from build123d import *

# Parameters (mm, degrees)
SKETCH_1_R          = 2.5
EXTRUDE_1_DEPTH     = 3
CUT_EXTRUDE_1_DEPTH = 2
SKETCH_3_R          = 1.5
EXTRUDE_2_DEPTH     = 10
FILLET_1_R          = 0.5
SKETCH_4_R          = 1.5
EXTRUDE_3_DEPTH     = 2


with BuildPart() as part:
    # 草图1 → 凸台-拉伸1 (new body)
    with BuildSketch(Plane(origin=(0, 0, 0), x_dir=(1, 0, 0), z_dir=(0, 1, 0))):
        with Locations(Location((0, 0, 0), (0, 0, 270))):
            Circle(SKETCH_1_R)
    extrude(amount=EXTRUDE_1_DEPTH)

    # 草图2 → 切除-拉伸1 (cut)
    with BuildSketch(Plane(origin=(0, 3, 0), x_dir=(1, 0, 0), z_dir=(0, 1, 0))):
        Polygon((0, 1.5), (-1.299038106, 0.75), (-1.299038106, -0.75), (0, -1.5), (1.299038106, -0.75), (1.299038106, 0.75), align=None)
    extrude(amount=-CUT_EXTRUDE_1_DEPTH, mode=Mode.SUBTRACT)

    # 草图3 → 凸台-拉伸2 (add)
    with BuildSketch(Plane.XZ):
        with Locations(Location((0, 0, 0), (0, 0, 270))):
            Circle(SKETCH_3_R)
    extrude(amount=EXTRUDE_2_DEPTH)

    # 圆角1
    fillet_1_edges = [part.edges().sort_by_distance(p)[0] for p in [
        (0, 0, -2.5),
        (0, 3, -2.5),
    ]]
    fillet(fillet_1_edges, radius=FILLET_1_R)

    # 草图4 → 凸台-拉伸3 (add)
    with BuildSketch(Plane.XZ.offset(10)):
        with Locations(Location((0, 0, 0), (0, 0, 270))):
            Circle(SKETCH_4_R)
    extrude(amount=EXTRUDE_3_DEPTH)


solid = part.part
Source: CAD feature listing. Evaluate the final solid. Frame: model axes, mm. A direction names the side the tool comes from. Round coordinates to 2 decimals unless told otherwise and drop trailing zeros. Loops run counter-clockwise (first coordinate to the right, second up) from the corner with the lowest first, then second, coordinate; pieces in that order, holes last. Notation, with made-up numbers: M 44,57 L 62,57 A23 ccw 62,65 Z; hole C 2.25,55 d3. An arc over 180 degrees is marked long. Return JSON: item names as keys, results as strings. Group by question number.
1. Section query A-A on z = 0. Output: boundary loops of the cut face in (x, y), and give its area (3 significant figures).
2. Pin query (flat end, axial travel): pin 1 (1.6 mm diameter, centred on y = 2.5, z = -0.5, fed in from +X); pin 2 (1 mm diameter, centred on x = 0.5, y = -6.5, fed in from +Z); pin 3 (1.5 mm diameter, centred on y = -7.5, z = 1.5, fed in from +X). Return the tip coordinate at first contact, or that it passes through.
3. Section query B-B on y = -3.25. Output: boundary loops of the cut face in (x, z).
4. Reachability of faces 5 (the face through (-0.66, 2.01, 1.12)), 6 (the face through (0.45, -5.92, -1.43)) from +Z, -Z, +X, -X, +Y, -Y: full face, straight path, thin tool, end or side. Return the list, or none.
5. Mould query, pull axis Z, two halves, no side actions, for faces 1 (the face through (1.299, 2, 0)), 2 (the face through (-2.44, 1.49, -0.54)), 3 (the face through (0, -12, 0)), 4 (the face through (0.66, 2.01, -1.12)). Classes: released by +Z, released by -Z, zero draft, split by the parting line, or undercut.
6. Material intervals for line 1 along Y through (x, z) = (1.1, 0.7); line 2 along Y through (x, z) = (-1, 1.5); line 3 along X through (y, z) = (-9.5, -1.3), sorted ascending. Write a range as from..to.
Checks:
{
 "1": {"outline": "M -2.5,0.5 A0.5 ccw -2,0 L -1.5,0 L -1.5,-12 L 1.5,-12 L 1.5,0 L 2,0 A0.5 ccw 2.5,0.5 L 2.5,2.5 A0.5 ccw 2,3 L 1.3,3 L 1.3,1 L -1.3,1 L -1.3,3 L -2,3 A0.5 ccw -2.5,2.5 Z", "area": "45.6 mm²"},
 "2": {"pin 1": "stops at x = 2.5", "pin 2": "stops at z = 1.5", "pin 3": "stops at x = 1.3"},
 "3": {"outline": "C 0,0 d3"},
 "4": {"face 5": "+Y", "face 6": "-Y"},
 "5": {"face 1": "undercut", "face 2": "split by the parting line", "face 3": "zero draft", "face 4": "undercut"},
 "6": {"line 1": "y = -12..1", "line 2": "y = 0..3", "line 3": "x = -0.75..0.75"}
}
